The drawing under review shows one solid part. Ordinate dimensions are in mm from its lowest x, y, z. Coordinates: 2 decimals unless noted, no trailing zeros. Order: outer loops, then holes, each group sorted by start corner. A loop starts at its lowest first (then second) coordinate and runs counter-clockwise, first axis right, second up. Notation, with made-up numbers: M -25.75,21 L 10.25,21 A26 cw 10.25,57 Z; hole C -24.75,-17 d3. An arc over 180 degrees is marked long. Answer as a JSON object with one key per item and string values.
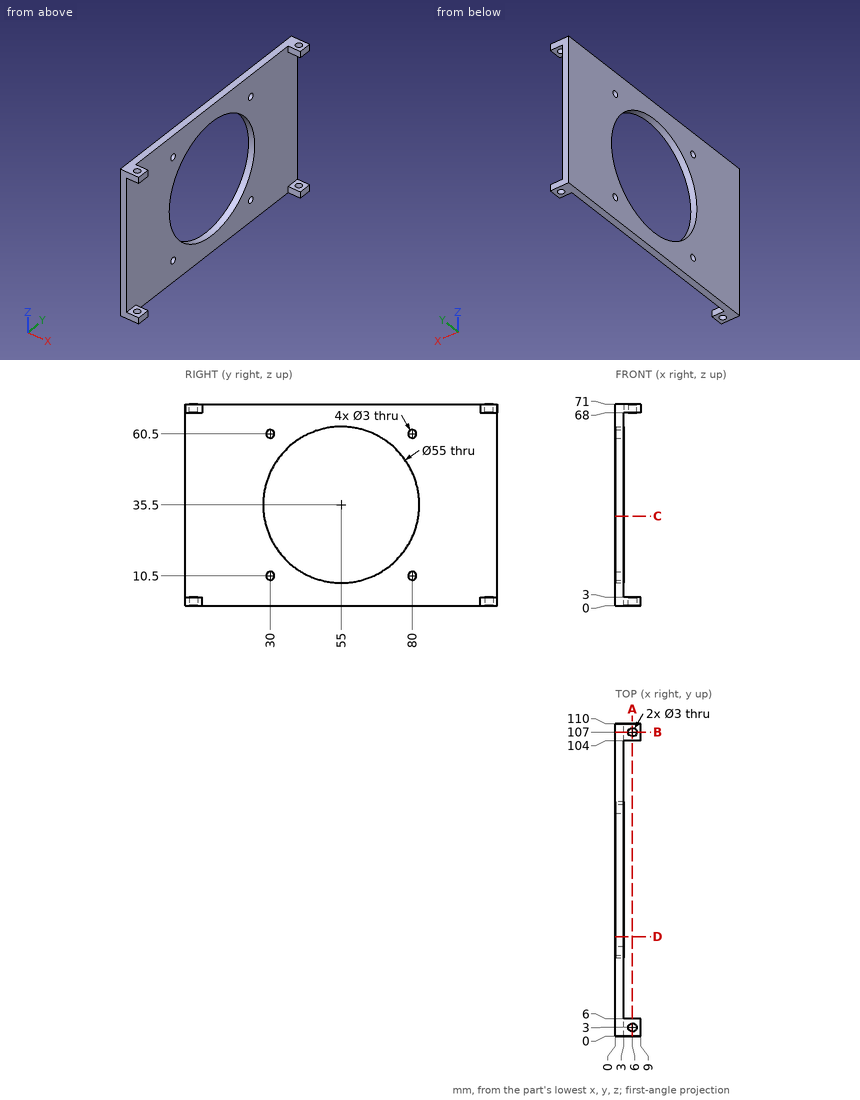
1) Add section D-D (y = 35). State the section outline as (x, z) points, and give its area (3 significant figures).
Taken from the geometry:
{"outline": "M 0,0 L 3,0 L 3,16.63 L 0,16.63 Z; M 0,54.37 L 3,54.37 L 3,71 L 0,71 Z", "area": "99.8 mm2"}
2) To check wall thickness, follow L1, parallel to Y at x = 6, z = 69.25; L2, parallel to X at y = 107, z = 69; L3, parallel to Z at x = 0.65, y = 30. State the ranges of each line that lie inside material, in increasing order.
Taken from the geometry:
{"L1": "y = 0 to 1.5, 4.5 to 6, 104 to 105.5, 108.5 to 110", "L2": "x = 0 to 4.5, 7.5 to 9", "L3": "z = 0 to 9, 12 to 24.04, 46.96 to 59, 62 to 71"}
3) Add section A-A (x = 6). Count the separate pieces of the cut face and the enclosed holes in it, and give its area (3 significant figures).
Taken from the geometry:
{"separate pieces": "8", "enclosed holes": "0", "area": "36.0 mm2"}
4) Add section B-B (y = 107). State the section outline as (x, z) points, and give its area (3 significant figures).
Taken from the geometry:
{"outline": "M 0,0 L 4.5,0 L 4.5,3 L 3,3 L 3,68 L 4.5,68 L 4.5,71 L 0,71 Z; M 7.5,0 L 9,0 L 9,3 L 7.5,3 Z; M 7.5,68 L 9,68 L 9,71 L 7.5,71 Z", "area": "231 mm2"}
5) Insertion check: pin 1 Ø1.8 at (x, y) = (6, 3) entering from +Z; pin 2 Ø1.5 at (y, z) = (11, 44.5) entering from -X; pin 3 Ø5 at (y, z) = (84.5, 53) entering from +X. Each pin has a flat end and moves straight along its axis. Give the tip position at first contact, or say it passes through.
Taken from the geometry:
{"pin 1": "passes through", "pin 2": "stops at x = 0", "pin 3": "stops at x = 3"}
6) Add section C-C (z = 31.5). State the section outline as (x, y) points.
Taken from the geometry:
{"outline": "M 0,0 L 3,0 L 3,27.79 L 0,27.79 Z; M 0,82.21 L 3,82.21 L 3,110 L 0,110 Z"}
